For this review, use the dimensioned drawing (mm, ordinates from the lowest corner) and the shaded views. A direction names the side the tool comes from. Round coordinates to 2 decimals unless told otherwise and drop trailing zeros. Write each loop counter-clockwise with the first axis right and the second up, starting at its lowest first coordinate (ties: lowest second). Pieces come first, ordered by that corner, then holes.
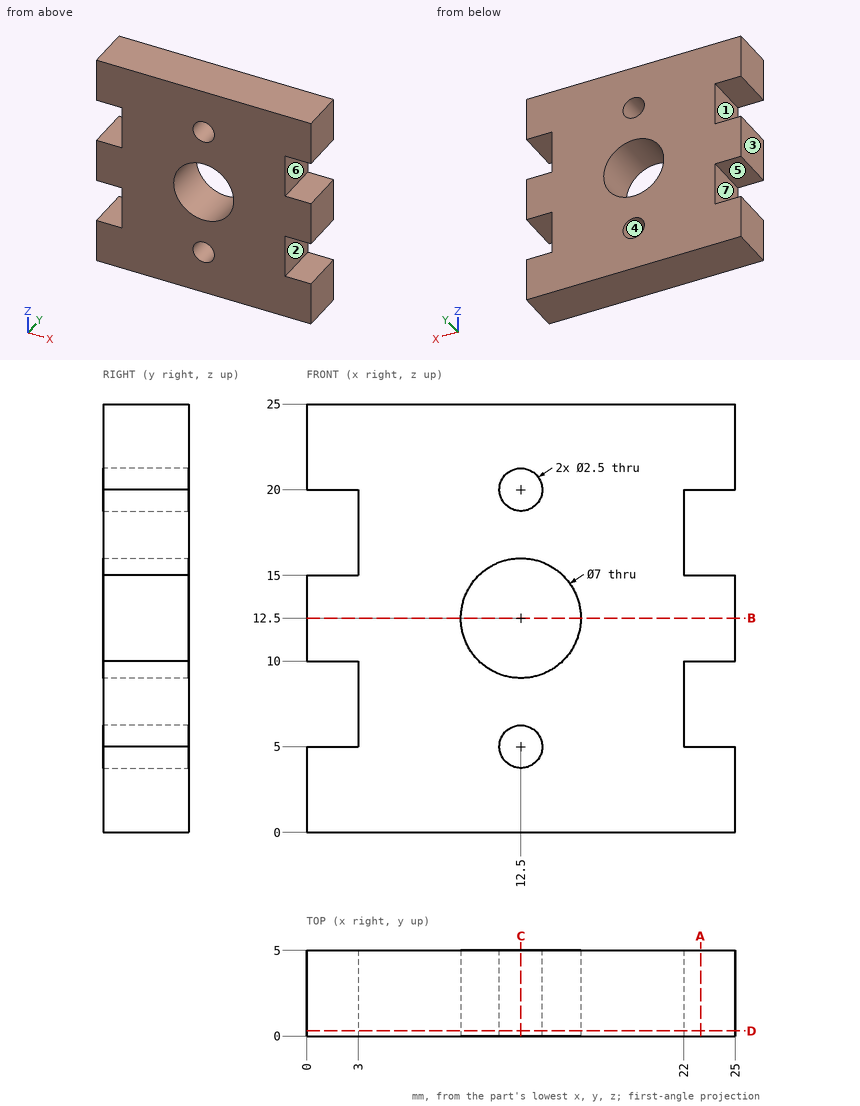
(1) For line 1 along X through (y, z) = (1.2, 12.5); line 2 along Z through (x, y) = (12.75, 2.35); line 3 along X through (y, z) = (2.55, 4.25), list the stretches that pass through material, from the lowest coordinate up.
Geometry check:
line 1: x = 0 to 9, 16 to 25
line 2: z = 0 to 3.78, 6.22 to 9.01, 15.99 to 18.78, 21.22 to 25
line 3: x = 0 to 11.5, 13.5 to 25
(2) We need section A-A, the plane x = 23. Give the boundary of the cut face in (y, z), and give its area (3 significant figures).
Geometry check:
outline: (0, 0) - (5, 0) - (5, 5) - (0, 5) - close; (0, 10) - (5, 10) - (5, 15) - (0, 15) - close; (0, 20) - (5, 20) - (5, 25) - (0, 25) - close
area: 75.0 mm2
(3) We need section C-C, the plane x = 12.5. Give the boundary of the cut face in (y, z).
Geometry check:
outline: (0, 0) - (5, 0) - (5, 3.75) - (0, 3.75) - close; (0, 6.25) - (5, 6.25) - (5, 9) - (0, 9) - close; (0, 16) - (5, 16) - (5, 18.75) - (0, 18.75) - close; (0, 21.25) - (5, 21.25) - (5, 25) - (0, 25) - close
(4) We need section B-B, the plane z = 12.5. Give the boundary of the cut face in (x, y).
Geometry check:
outline: (0, 0) - (9, 0) - (9, 5) - (0, 5) - close; (16, 0) - (25, 0) - (25, 5) - (16, 5) - close
(5) For the marked faces 1, 2 and 3, list the 3-axis set-ups (+Z, -Z, +X, -X, +Y, -Y) from which the entire face can be reached by the end or side of a thin tool; tool diameter is ignored.
Geometry check:
face 1: -X, +Y, -Y
face 2: +X, +Y, -Y
face 3: +Z, -Z, -X, +Y, -Y
(6) For pin 1 Ø2.5 at (y, z) = (2, 17) entering from +X, flat-tipped, find the tip position at first contact; note if it passes through.
Geometry check:
pin 1: stops at x = 22
(7) We need section D-D, the plane y = 0.3. Give the boundary of the cut face in (x, z).
Geometry check:
outline: (0, 0) - (25, 0) - (25, 5) - (22, 5) - (22, 10) - (25, 10) - (25, 15) - (22, 15) - (22, 20) - (25, 20) - (25, 25) - (0, 25) - (0, 20) - (3, 20) - (3, 15) - (0, 15) - (0, 10) - (3, 10) - (3, 5) - (0, 5) - close; hole circle Ø7 at (12.5, 12.5); hole circle Ø2.5 at (12.5, 5); hole circle Ø2.5 at (12.5, 20)
(8) Mouldability with a two-part tool opening along X and no side actions: class the marked faces 4, 5, 6 and 7 as pulls with the +X half, pulls with the -X half, needs draft (parallel to the pull), parting line crosses it, or undercut.
Geometry check:
face 4: undercut
face 5: needs draft
face 6: pulls with the +X half
face 7: pulls with the -X half
